Verification items for this drawing (mm, ordinates from the low corner). Give positions to 0.01 mm unless a question says otherwise; leave off trailing zeros. Order: outer loops, then holes, each group sorted by start corner. A loop starts at its lowest first (then second) coordinate and runs counter-clockwise, first axis right, second up.
(1) Sectioned sample at A-A on y = 91.44. Record the cut outline in (x, z) (1 decimal), plus the area to 3 significant figures.
(2) Scan lines: L1, parallel to Y at x = 12.7, z = 1.25; L2, parallel to Y at x = 72.39, z = 2; L3, parallel to Y at x = 33, z = 1.6. Record each from-to range of solid material in increasing order.
(3) Sectioned sample at D-D on z = 0.6. Record the cut outline in (x, y).
(4) Sectioned sample at C-C on x = 12.7. Record the cut outline in (y, z) (1 decimal).
(5) Gauge pin test, flat end, axial feed: pin 1 (1 mm diameter, centred on y = 67.5, z = 2, fed in from +X). Record the tip position at first contact, or that the pin passes through.
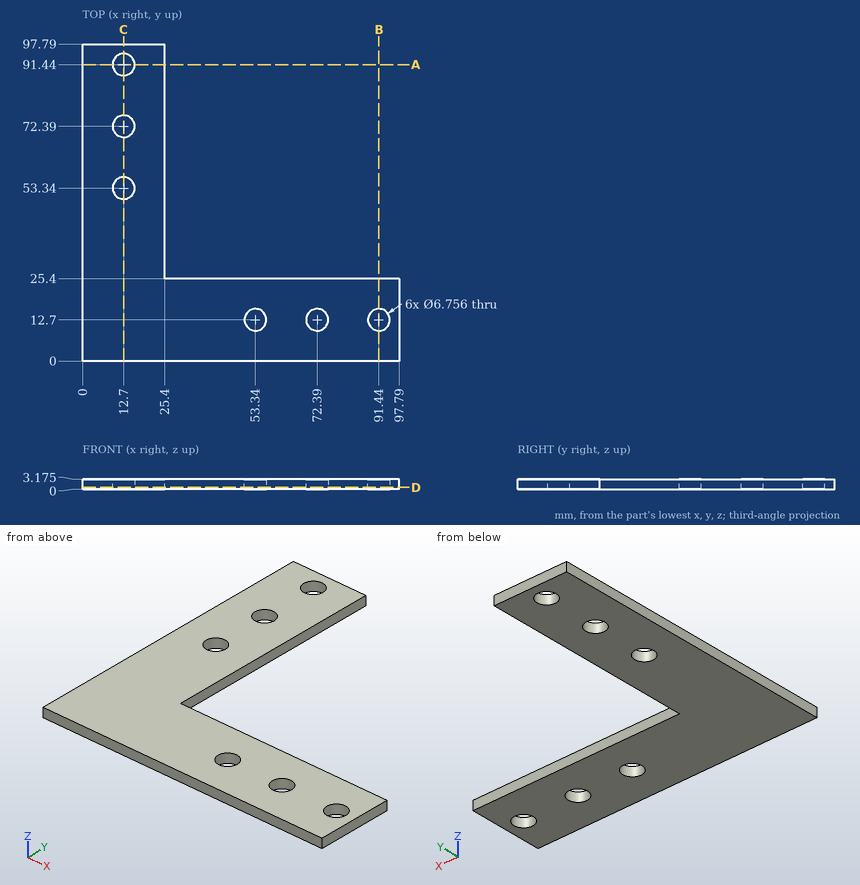
Ans:
1. outline: (0, 0) - (9.3, 0) - (9.3, 3.2) - (0, 3.2) - close; (16.1, 0) - (25.4, 0) - (25.4, 3.2) - (16.1, 3.2) - close
1. area: 59.2 mm2
2. L1: y = 0 to 49.96, 56.72 to 69.01, 75.77 to 88.06, 94.82 to 97.79
2. L2: y = 0 to 9.32, 16.08 to 25.4
2. L3: y = 0 to 25.4
3. outline: (0, 0) - (97.79, 0) - (97.79, 25.4) - (25.4, 25.4) - (25.4, 97.79) - (0, 97.79) - close; hole circle Ø6.76 at (12.7, 53.34); hole circle Ø6.76 at (12.7, 72.39); hole circle Ø6.76 at (12.7, 91.44); hole circle Ø6.76 at (53.34, 12.7); hole circle Ø6.76 at (72.39, 12.7); hole circle Ø6.76 at (91.44, 12.7)
4. outline: (0, 0) - (50, 0) - (50, 3.2) - (0, 3.2) - close; (56.7, 0) - (69, 0) - (69, 3.2) - (56.7, 3.2) - close; (75.8, 0) - (88.1, 0) - (88.1, 3.2) - (75.8, 3.2) - close; (94.8, 0) - (97.8, 0) - (97.8, 3.2) - (94.8, 3.2) - close
5. pin 1: stops at x = 25.4
